from build123d import *

# Parameters (mm, degrees)
SKETCH1_W           = 60
SKETCH1_H           = 60
BOSS_EXTRUDE1_DEPTH = 7.5
SKETCH3_R           = 10
BOSS_EXTRUDE2_DEPTH = 5


with BuildPart() as part:
    # Sketch1 → Boss-Extrude1 (new body, symmetric)
    with BuildSketch(Plane.XY):
        Rectangle(SKETCH1_W, SKETCH1_H)
    extrude(amount=BOSS_EXTRUDE1_DEPTH, both=True)

    # Sketch3 → Boss-Extrude2 (add, symmetric)
    with BuildSketch(Plane(origin=(0, 0, 0), x_dir=(0, 0, -1), z_dir=(1, 0, 0))):
        with BuildLine():
            Line((-7.5, 20), (-27.5, 20))
            ThreePointArc((-27.5, 20), (-47.5, 0), (-27.5, -20))
            Line((-27.5, -20), (-7.5, -20))
            Line((-7.5, -20), (-7.5, 20))
        make_face()
        with Locations((-27.5, 0)):
            Circle(SKETCH3_R, mode=Mode.SUBTRACT)
    extrude(amount=BOSS_EXTRUDE2_DEPTH, both=True)


solid = part.part
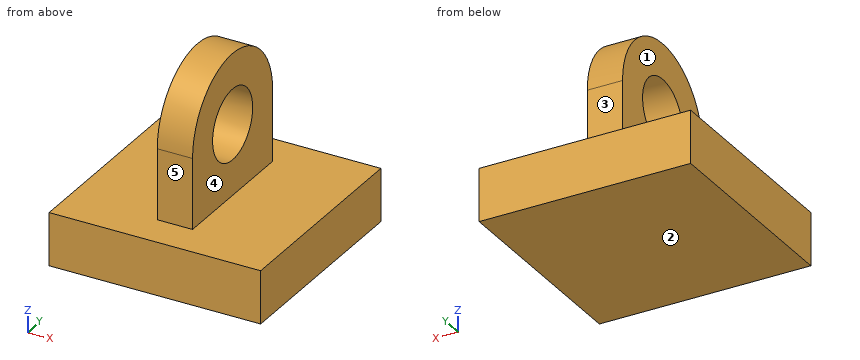
CAD build for the part. Positions are in the model's coordinates, mm. Face numbers are marked on the shaded views. A direction names the side the tool comes from. Round coordinates to 2 decimals unless told otherwise and drop trailing zeros. Order: outer loops, then holes, each group sorted by start corner. A loop starts at its lowest first (then second) coordinate and runs counter-clockwise, first axis right, second up. Notation, with made-up numbers: (-36.5, 7.5) -> (-17.5, 7.5) arc R19 ccw to (-17.5, 11.5) -> close; hole circle Ø9 at (11.5, -36). An arc over 180 degrees is marked (long way). Write item = value, one per line. Start each with the question number.
(1) Cut at A-A, the plane y = 0. List the corners of the cut face in (x, z).
(2) Probe line 1 (Y direction, x = -0.25, z = 27.5); line 2 (X direction, y = -19, z = 27); line 3 (Z direction, x = -4, y = -20.5). List the from-to ranges inside material, lowest first. Write a range as [from, to].
(3) Which spindle directions (+Z, -Z, +X, -X, +Y, -Y) get a long thin tool onto all of the face, cutting with end or side? Do the marked faces 1, 2, 3, 4 and 5. Say none if no direction does.
(4) Cut at B-B, the plane z = 34. List the corners of the cut face in (x, y), then the cut area to 3 significant figures.
(5) Cut at C-C, the plane y = 25.5. List the corners of the cut face in (x, z), then the cut area to 3 significant figures.
(6) Pin check, flat tips, straight feed: P1, Ø20, axis at y = 9.5, z = 24.5, coming from the -X side; P2, Ø11, axis at x = -1.5, z = 14.5, coming from the -Y side; P3, Ø5, axis at x = -1, z = 13.5, coming from the +Y side. Stop position of each tip, or through.
Model answer:
q1.outline = (-30, -7.5) -> (30, -7.5) -> (30, 7.5) -> (5, 7.5) -> (5, 17.5) -> (-5, 17.5) -> (-5, 7.5) -> (-30, 7.5) -> close; (-5, 37.5) -> (5, 37.5) -> (5, 47.5) -> (-5, 47.5) -> close
q2.line_1 = [-20, -10], [10, 20]
q2.line_2 = [-5, 5]
q2.line_3 = [-7.5, 7.5]
q3.face_1 = +Z, -X, +Y, -Y
q3.face_2 = -Z, +X, -X, +Y, -Y
q3.face_3 = +Z, +X, -X, +Y
q3.face_4 = +Z, +X, +Y, -Y
q3.face_5 = +Z, +X, -X, -Y
q4.outline = (-5, -18.91) -> (5, -18.91) -> (5, -7.6) -> (-5, -7.6) -> close; (-5, 7.6) -> (5, 7.6) -> (5, 18.91) -> (-5, 18.91) -> close
q4.area = 226 mm2
q5.outline = (-30, -7.5) -> (30, -7.5) -> (30, 7.5) -> (-30, 7.5) -> close
q5.area = 900 mm2
q6.P1 = -5
q6.P2 = -20
q6.P3 = 20
